Geometry: final body of the model. Coordinates: model frame, mm. Coordinates: 2 decimals unless noted, no trailing zeros. Order: outer loops, then holes, each group sorted by start corner. A loop starts at its lowest first (then second) coordinate and runs counter-clockwise, first axis right, second up. Notation, with made-up numbers: (19, 66.25) -> (28, 66.25) arc R31 cw to (28, 103.25) -> close; hole circle Ø8 at (-35.75, 7.25). An arc over 180 degrees is marked (long way). Use one line per item in the form item = value.
```python
from build123d import *

# Parameters (mm, degrees)
SKETCH_1_W          = 89
SKETCH_1_H          = 62
EXTRUDE_1_DEPTH     = 5
CUT_EXTRUDE_START   = -5.000001
SKETCH_2_W          = 114.345269922
SKETCH_2_H          = 82.741202996
CUT_EXTRUDE_2_DEPTH = 5.000002
FILLET_1_R          = 5


with BuildPart() as part:
    # 草图1 → 凸台-拉伸1 (new body)
    with BuildSketch(Plane(origin=(0, 0, 0), x_dir=(1, 0, 0), z_dir=(0, 1, 0))):
        with Locations((-7.7, -10.288888889)):
            Rectangle(SKETCH_1_W, SKETCH_1_H)
    extrude(amount=EXTRUDE_1_DEPTH)

    # 草图2 → 切除-拉伸2 (cut)
    with BuildSketch(Plane(origin=(0, 5, 0), x_dir=(1, 0, 0), z_dir=(0, 1, 0)).offset(CUT_EXTRUDE_START)):
        with Locations((-11.341983823, -7.488413354)):
            Rectangle(SKETCH_2_W, SKETCH_2_H)
        with BuildLine():
            Line((-28.520508076, 20.711111111), (13.120508076, 20.711111111))
            ThreePointArc((13.120508076, 20.711111111), (23.620508076, 17.897644591), (31.307041555, 10.211111111))
            ThreePointArc((31.307041555, 10.211111111), (36.8, -10.288888889), (31.307041555, -30.788888889))
            ThreePointArc((31.307041555, -30.788888889), (23.620508076, -38.475422368), (13.120508076, -41.288888889))
            Line((13.120508076, -41.288888889), (-28.520508076, -41.288888889))
            ThreePointArc((-28.520508076, -41.288888889), (-39.020508076, -38.475422368), (-46.707041555, -30.788888889))
            ThreePointArc((-46.707041555, -30.788888889), (-52.2, -10.288888889), (-46.707041555, 10.211111111))
            ThreePointArc((-46.707041555, 10.211111111), (-39.020508076, 17.897644591), (-28.520508076, 20.711111111))
        make_face(mode=Mode.SUBTRACT)
    extrude(amount=CUT_EXTRUDE_2_DEPTH, mode=Mode.SUBTRACT)

    # 圆角1
    fillet_1_edges = [part.edges().sort_by_distance(p)[0] for p in [
        (36.8, 5, 10.288888889),
        (23.620508076, 5, 38.475422368),
        (-7.7, 5, 41.288888889),
        (-39.020508076, 5, 38.475422368),
        (-52.2, 5, 10.288888889),
        (-39.020508076, 5, -17.897644591),
        (-7.7, 5, -20.711111111),
        (23.620508076, 5, -17.897644591),
    ]]
    fillet(fillet_1_edges, radius=FILLET_1_R - 0.0001)  # a hair under: the kernel refuses the full size


solid = part.part
```
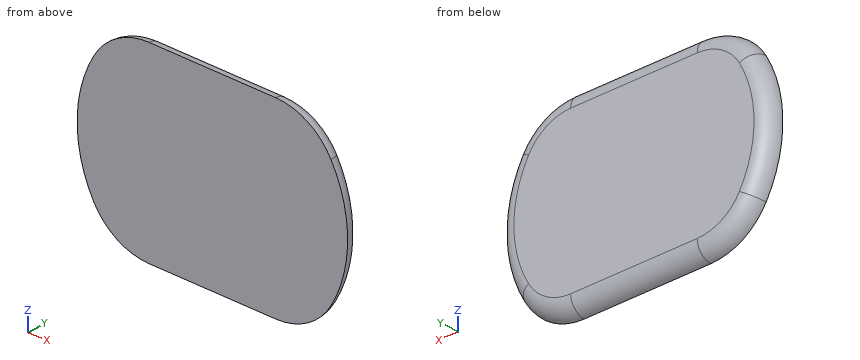
1) Section B-B, the plane y = 1.4. Output: boundary loops of the cut face in (x, z).
Results found:
outline = (-46.53, -10.11) arc R20.8 ccw to (-28.52, -20.51) -> (13.12, -20.51) arc R20.8 ccw to (31.13, -10.11) arc R40.8 ccw to (31.13, 30.69) arc R20.8 ccw to (13.12, 41.09) -> (-28.52, 41.09) arc R20.8 ccw to (-46.53, 30.69) arc R40.8 ccw to start
2) Contact query for a flat-ended pin moving along its axis: P1, Ø1, axis at x = -39.5, y = 3, coming from the +Z side. Output: stop coordinate, or through.
Results found:
P1 = 37.52
3) Material intervals for probe 1 along X at (y, z) = (3.45, 5.5); probe 2 along Z at (x, y) = (-18.5, 3.45); probe 3 along X at (y, z) = (1.2, 2), sorted ascending. Write a range as from..to.
Results found:
probe_1 = -50.53..35.13
probe_2 = -19.33..39.91
probe_3 = -51.2..35.8
